```python
from build123d import *

# Parameters (mm, degrees)
SKETCH1_W           = 200
SKETCH1_H           = 150
BOSS_EXTRUDE1_DEPTH = 5
BOSS_EXTRUDE2_DEPTH = 35
SKETCH4_W           = 155
SKETCH4_H           = 5
BOSS_EXTRUDE3_DEPTH = 8
SKETCH5_W           = 155
SKETCH5_H           = 5
BOSS_EXTRUDE4_DEPTH = 8


with BuildPart() as part:
    # Sketch1 → Boss-Extrude1 (new body)
    with BuildSketch(Plane(origin=(0, 0, 0), x_dir=(1, 0, 0), z_dir=(0, 1, 0))):
        with Locations((100, -75)):
            Rectangle(SKETCH1_W, SKETCH1_H)
    extrude(amount=BOSS_EXTRUDE1_DEPTH)

    # Sketch2 → Boss-Extrude2 (add)
    with BuildSketch(Plane(origin=(0, 5, 0), x_dir=(1, 0, 0), z_dir=(0, 1, 0))):
        Polygon((0, -150), (-5, -150), (-5, 0), (-5, 5), (205, 5), (205, 0), (205, -150), (200, -150), (200, 0), (0, 0), align=None)
    extrude(amount=-BOSS_EXTRUDE2_DEPTH)

    # Sketch4 → Boss-Extrude3 (add)
    with BuildSketch(Plane(origin=(205, 0, 0), x_dir=(0, 0, -1), z_dir=(1, 0, 0))):
        with Locations((-72.5, -27.5)):
            Rectangle(SKETCH4_W, SKETCH4_H)
    extrude(amount=BOSS_EXTRUDE3_DEPTH)

    # Sketch5 → Boss-Extrude4 (add)
    with BuildSketch(Plane.ZY.offset(5)):
        with Locations((72.5, -27.5)):
            Rectangle(SKETCH5_W, SKETCH5_H)
    extrude(amount=BOSS_EXTRUDE4_DEPTH)


solid = part.part
```
Check sheet for the modelled part. Datum: model origin and axes. Units: mm. A direction names the side the tool comes from. Coordinates: 2 decimals unless noted, no trailing zeros. Order: outer loops, then holes, each group sorted by start corner. A loop starts at its lowest first (then second) coordinate and runs counter-clockwise, first axis right, second up. Notation, with made-up numbers: (-12, -35.75) -> (26, -35.75) arc R35 cw to (26, -1.75) -> close; hole circle Ø8 at (78.25, -29). An arc over 180 degrees is marked (long way). Write item = value, one per line. Start each with the question number.
1) Mould release check, pull along X, two halves, no side actions. Record for faces 1 (the flat face through (125.6, 0.4, 150)), 2 (the flat face through (205, -10, 74)), 3 (the flat face through (-5, -10, 71)), 4 (the flat face through (101, -15, 0)): +X half, -X half, draft (parallel to the pull), parting line (faces both ways), or undercut.
2) Cross-section at B-B (x = 104). Enter the section's corners in (y, z).
3) Cross-section at C-C (z = 15). Enter the section's corners in (x, y).
4) Material ranges on L1, parallel to X at y = -9.5, z = 73; L2, parallel to X at y = -28, z = 81; L3, parallel to Y at x = 14.5, z = 14, recorded low to high.
5) Access from +Z, -Z, +X, -X, +Y, -Y to the whole of each face (thin tool, end or side, straight path). Record for faces 5 (the flat face through (213, -27, 74)), 6 (the flat face through (-9, -25, 71)), 7 (the flat face through (209, -25, 74)), 8 (the flat face through (200, -15, 76)).
6) Go/stop test with flat-tipped pins: P1, Ø4, axis at y = -20, z = 105.5, coming from the +X side; P2, Ø10, axis at x = 64, z = 26.5, coming from the -Y side; P3, Ø1, axis at y = -18.5, z = 76.5, coming from the -X side. Record where each tip stops, or that it passes through.
7) Cross-section at A-A (y = -3). Enter the section's corners in (x, z), then the cut area to 3 significant figures.
Ans:
q1.face_1 = draft
q1.face_2 = +X half
q1.face_3 = -X half
q1.face_4 = undercut
q2.outline = (-30, -5) -> (5, -5) -> (5, 150) -> (0, 150) -> (0, 0) -> (-30, 0) -> close
q3.outline = (-13, -30) -> (0, -30) -> (0, 0) -> (200, 0) -> (200, -30) -> (213, -30) -> (213, -25) -> (205, -25) -> (205, 5) -> (-5, 5) -> (-5, -25) -> (-13, -25) -> close
q4.L1 = -5 to 0, 200 to 205
q4.L2 = -13 to 0, 200 to 213
q4.L3 = 0 to 5
q5.face_5 = +Z, -Z, +X, +Y, -Y
q5.face_6 = +Z, -Z, -X, +Y
q5.face_7 = +Z, -Z, +X, +Y
q5.face_8 = +Z, -Y
q6.P1 = 205
q6.P2 = 0
q6.P3 = -5
q7.outline = (-5, -5) -> (205, -5) -> (205, 150) -> (200, 150) -> (200, 0) -> (0, 0) -> (0, 150) -> (-5, 150) -> close
q7.area = 2,550 mm²
